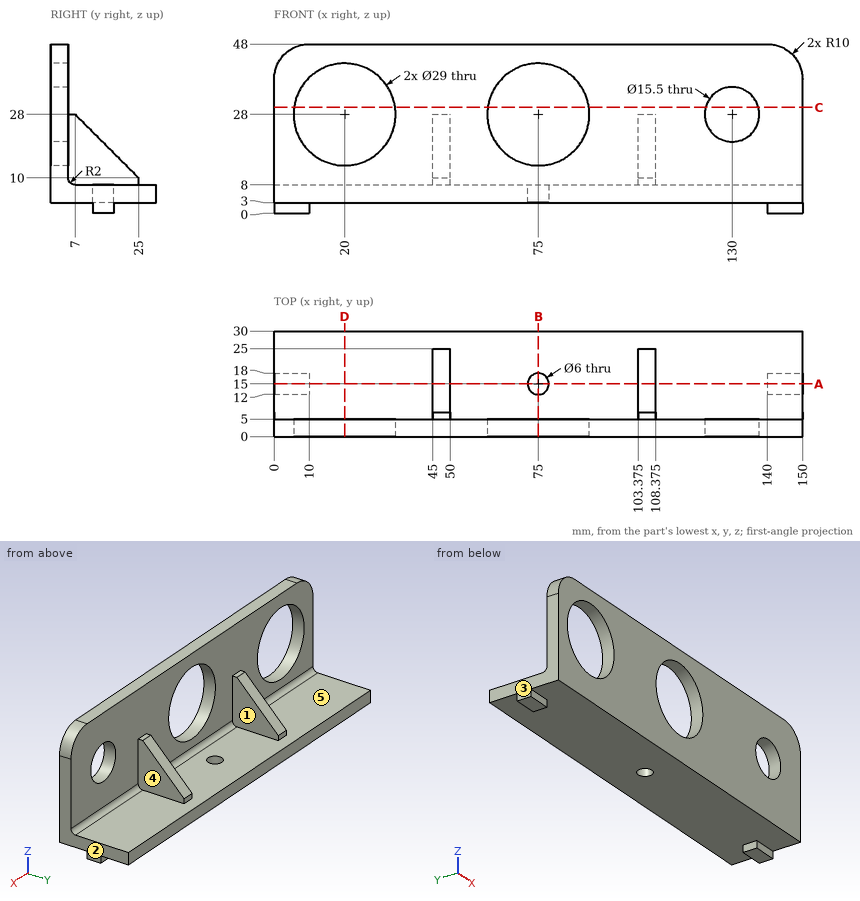
Verification items for this drawing (mm, ordinates from the low corner). A direction names the side the tool comes from. Round coordinates to 2 decimals unless told otherwise and drop trailing zeros. Order: outer loops, then holes, each group sorted by start corner. A loop starts at its lowest first (then second) coordinate and runs counter-clockwise, first axis right, second up. Notation, with made-up numbers: M 48.5,80 L 107.5,80 A26 ccw 107.5,94 Z; hole C 55.5,45 d2. An arc over 180 degrees is marked long. Answer in a Markdown table with one row per item. Add a question column.
Item 1: Depth check by flat-ended pin: pin 1 Ø5 at (y, z) = (14.5, 20.5) entering from -X; pin 2 Ø1.5 at (x, z) = (7.5, 1.5) entering from -Y; pin 3 Ø5 at (x, z) = (32.5, 39) entering from +Y; pin 4 Ø12.5 at (x, z) = (130, 28) entering from +Y. Enter the tip coordinate at first touch or a pass-through.
Item 2: Sectioned sample at A-A, the plane y = 15. Enter the section's corners in (x, z) (3 decimals).
Item 3: Sectioned sample at B-B, the plane x = 75. Enter the section's corners in (y, z), plus the area to 3 significant figures.
Item 4: Set-up check for the marked faces 1 and 2: record each of +Z, -Z, +X, -X, +Y, -Y from which the full face is reachable in a straight line by a thin tool's end or side.
Item 5: Material ranges on L1, parallel to Y at x = 75, z = 5; L2, parallel to Z at x = 130, y = 2.8; L3, parallel to Z at x = 75, y = 2.55, recorded low to high. Write a range as [from, to].
Item 6: Sectioned sample at C-C, the plane z = 30. Enter the section's corners in (x, y), plus the area to 3 significant figures.
Item 7: Sectioned sample at D-D, the plane x = 20. Enter the section's corners in (y, z).
Item 8: Draft check along X on the marked faces 3, 4 and 5. Enter one of: released by +X, released by -X, zero draft, split by the parting line, or undercut.
Filled in:
| question | item | result |
|---|---|---|
| 1 | pin 1 | stops at x = 45 |
| 1 | pin 2 | stops at y = 12 |
| 1 | pin 3 | stops at y = 5 |
| 1 | pin 4 | passes through |
| 2 | outline | M 0,0 L 10,0 L 10,3 L 72,3 L 72,8 L 50,8 L 50,20 L 45,20 L 45,8 L 0,8 Z; M 78,3 L 140,3 L 140,0 L 150,0 L 150,8 L 108.375,8 L 108.375,20 L 103.375,20 L 103.375,8 L 78,8 Z |
| 3 | outline | M 0,3 L 12,3 L 12,8 L 7,8 A2 cw 5,10 L 5,13.5 L 0,13.5 Z; M 0,42.5 L 5,42.5 L 5,48 L 0,48 Z; M 18,3 L 30,3 L 30,8 L 18,8 Z |
| 3 | area | 176 mm² |
| 4 | face 1 | +Z, +Y |
| 4 | face 2 | +Z, -Z, +X, +Y, -Y |
| 5 | L1 | y = [0, 12], [18, 30] |
| 5 | L2 | z = [3, 20.25], [35.75, 48] |
| 5 | L3 | z = [3, 13.5], [42.5, 48] |
| 6 | outline | M 0,0 L 5.64,0 L 5.64,5 L 0,5 Z; M 34.36,0 L 60.64,0 L 60.64,5 L 34.36,5 Z; M 89.36,0 L 122.51,0 L 122.51,5 L 89.36,5 Z; M 137.49,0 L 150,0 L 150,5 L 137.49,5 Z |
| 6 | area | 388 mm² |
| 7 | outline | M 0,3 L 30,3 L 30,8 L 7,8 A2 cw 5,10 L 5,13.5 L 0,13.5 Z; M 0,42.5 L 5,42.5 L 5,48 L 0,48 Z |
| 8 | face 3 | released by -X |
| 8 | face 4 | released by +X |
| 8 | face 5 | undercut |
